```python
from build123d import *

# Parameters (mm, degrees)
SKETCH_1_W      = 6
SKETCH_1_H      = 30
EXTRUDE_1_DEPTH = 15
CHAMFER_1_SIZE  = 5


with BuildPart() as part:
    # Эскиз1 → Бобышка-Вытянуть1 (new body)
    with BuildSketch(Plane(origin=(0, 0, 0), x_dir=(1, 0, 0), z_dir=(0, 1, 0))):
        with Locations((3, 15)):
            Rectangle(SKETCH_1_W, SKETCH_1_H)
    extrude(amount=EXTRUDE_1_DEPTH)

    # Фаска1
    chamfer_1_edges = [part.edges().sort_by_distance(p)[0] for p in [
        (3, 15, 0),
    ]]
    chamfer(chamfer_1_edges, length=CHAMFER_1_SIZE)


solid = part.part
```
Could you check a few things on this model? Use its own coordinates, in mm. Give positions to 0.01 mm unless a question says otherwise; leave off trailing zeros. Loops run counter-clockwise (first coordinate to the right, second up) from the corner with the lowest first, then second, coordinate; pieces in that order, holes last. Notation, with made-up numbers: (-36, -10.75) - (-5, -10.75) arc R14 ccw to (-5, -6.75) - close; hole circle Ø8 at (-24.75, 69). An arc over 180 degrees is marked (long way). Use one line per item in the form item = value.
1. I'm going to push a flat-ended pin straight in: pin 1 Ø2 at (x, z) = (2.5, -3.5) entering from +Y. Where does the tip first touch, or does it pass through?
Response values:
pin_1 = 14.5
2. I need wall thicknesses on probe 1 along Y at (x, z) = (5.15, -3.75); probe 2 along Y at (x, z) = (0.35, -2.5); probe 3 along Z at (x, y) = (2.45, 11.75). Which ranges of each line are inside material? Lowest first, please.
Response values:
probe_1 = 0 to 13.75
probe_2 = 0 to 12.5
probe_3 = -30 to -1.75
3. I want a section at B-B (z = -3.25). Please give me the cut outline in (x, y), and give its area (3 significant figures).
Response values:
outline = (0, 0) - (6, 0) - (6, 13.25) - (0, 13.25) - close
area = 79.5 mm²
4. I want a section at C-C (y = 11). Please give me the cut outline in (x, z).
Response values:
outline = (0, -30) - (6, -30) - (6, -1) - (0, -1) - close
5. I want a section at A-A (x = 5.05). Please give me the cut outline in (y, z).
Response values:
outline = (0, -30) - (15, -30) - (15, -5) - (10, 0) - (0, 0) - close
